Design review of the part built by this model. Coordinates are the model's own, in mm. A direction names the side the tool comes from. Give positions to 0.01 mm unless a question says otherwise; leave off trailing zeros. Order: outer loops, then holes, each group sorted by start corner. A loop starts at its lowest first (then second) coordinate and runs counter-clockwise, first axis right, second up. Notation, with made-up numbers: M 86,-18.5 L 106,-18.5 A29 cw 106,17.5 Z; hole C 14.25,17 d8. An arc over 180 degrees is marked long. Put each result on its own line as item: value. Start each with the question number.
from build123d import *

# Parameters (mm, degrees)
F0_R     = 31.75
F0_R_2   = 30.1625
F1_DEPTH = 63.5
F0_R_3   = 25.4
F2_DEPTH = 76.2
F0_R_4   = 19.05
F3_DEPTH = 50.8
F0_R_5   = 15.875
F4_DEPTH = 50.8
F5_DEPTH = 47.625
F8_SIZE  = 0.508
F9_SIZE  = 0.508
F10_SIZE = 8.89
F11_SIZE = 8.89
F13_R    = 12.7
F14_R    = 6.35


with BuildPart() as f1:
    # F0 (on Top) → F1 (new body)
    with BuildSketch(Plane.XY):
        Circle(F0_R)
        Circle(F0_R_2, mode=Mode.SUBTRACT)
    extrude(amount=F1_DEPTH)

    # F0 (on Top) → F2 (join)
    with BuildSketch(Plane.XY):
        Circle(F0_R_2)
        Circle(F0_R_3, mode=Mode.SUBTRACT)
    extrude(amount=F2_DEPTH)

    # F0 (on Top) → F3 (join)
    with BuildSketch(Plane.XY):
        Circle(F0_R_3)
        Circle(F0_R_4, mode=Mode.SUBTRACT)
    extrude(amount=F3_DEPTH)

    # F0 (on Top) → F4 (join)
    with BuildSketch(Plane.XY):
        Circle(F0_R_4)
        Circle(F0_R_5, mode=Mode.SUBTRACT)
    extrude(amount=F4_DEPTH)

    # F0 (on Top) → F5 (cut)
    with BuildSketch(Plane.XY):
        Circle(F0_R_4)
        Circle(F0_R_5, mode=Mode.SUBTRACT)
    extrude(amount=F5_DEPTH, mode=Mode.SUBTRACT)

    # F8
    f8_edges = [f1.edges().sort_by_distance(p)[0] for p in [
        (-19.05, 0, 0),
        (-31.75, 0, 63.5),
        (-30.1625, 0, 76.2),
        (-25.4, 0, 76.2),
    ]]
    chamfer(f8_edges, length=F8_SIZE)

    # F9
    f9_edges = [f1.edges().sort_by_distance(p)[0] for p in [
        (-15.875, 0, 50.8),
        (-15.875, 0, 47.625),
    ]]
    chamfer(f9_edges, length=F9_SIZE)

    # F10
    f10_edges = [f1.edges().sort_by_distance(p)[0] for p in [
        (-31.75, 0, 0),
    ]]
    chamfer(f10_edges, length=F10_SIZE)

    # F11
    f11_edges = [f1.edges().sort_by_distance(p)[0] for p in [
        (-31.75, 0, 8.89),
    ]]
    chamfer(f11_edges, length=F11_SIZE)

    # F13
    f13_edges = [f1.edges().sort_by_distance(p)[0] for p in [
        (-31.749992, 0, 17.78),
    ]]
    fillet(f13_edges, radius=F13_R)

    # F14
    f14_edges = [f1.edges().sort_by_distance(p)[0] for p in [
        (-25.463814, 0, 2.603821),
    ]]
    fillet(f14_edges, radius=F14_R)


solid = f1.part
1. To check wall thickness, follow probe 1 along Y at (x, z) = (0, 68.5); probe 2 along Y at (x, z) = (0, 58); probe 3 along Z at (x, y) = (-7.5, -15) (3 decimals). State the ranges of each line that lie inside material, in increasing order.
2. Machinability: for faces 4 (the cylindrical face through (-3.441, -15.497, 49.197)), 5 (the cylindrical face through (-15.12, -11.59, 23.74)), 6 (the flat face through (0, -17, 50.8)), which of the approach directions +Z, -Z, +X, -X, +Y, -Y give a long, thin tool a straight path to every point of the face, cutting with its end or side? Answer none if there is none.
3. The part is to be moulded in two halves that separate along X. For faces 1 (the cylindrical face through (-30.133, 1.326, 69.511)), 2 (the flat face through (-16, 26, 63.5)), 3 (the cylindrical face through (-5.506, -24.796, 63.072)), say which applies: +X half, -X half, draft (parallel to the pull), parting line (faces both ways), or undercut.
4. Consider section A-A on z = 53.5. Give the boundary of the cut face in (x, y).
5. Insertion check: pin 1 (19 mm diameter, centred on x = 0, y = 0, fed in from +Z); pin 2 (6 mm diameter, centred on x = 21.5, z = 47, fed in from +Y); pin 3 (1 mm diameter, centred on x = -12, z = 56.5, fed in from -Y); pin 4 (1 mm diameter, centred on y = -9, z = 54, fed in from -X). Each pin has a flat end and moves straight along its axis. Give the tip position at first contact, or say it passes through.
Returned:
1. probe 1: y = -30.16 to -25.4, 25.4 to 30.16
1. probe 2: y = -31.75 to -25.4, 25.4 to 31.75
1. probe 3: z = 47.625 to 50.8
2. face 4: +Z, -Z
2. face 5: -Z
2. face 6: +Z
3. face 1: parting line
3. face 2: draft
3. face 3: undercut
4. outline: C 0,0 d63.5; hole C 0,0 d50.8
5. pin 1: passes through
5. pin 2: stops at y = 25.8
5. pin 3: stops at y = -29.59
5. pin 4: stops at x = -30.59
